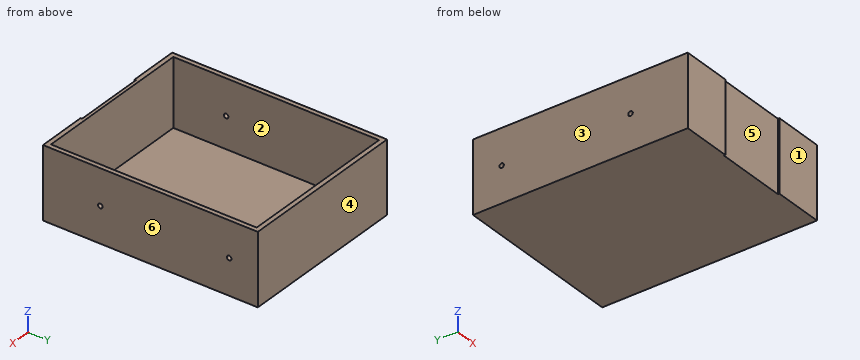
```python
from build123d import *

# Parameters (mm, degrees)
F0_W     = 113.645
F0_H     = 3.18
F0_W_2   = 3.175
F0_H_2   = 143.64
F0_W_3   = 3.18
F1_DEPTH = 50
F2_W     = 113.64
F2_H     = 143.64
F3_DEPTH = 47
F5_DEPTH = 120.001
F6_W     = 50
F6_H     = 50
F7_DEPTH = 1


with BuildPart() as f1:
    # F0 (on Top) → F1 (new body)
    with BuildSketch(Plane.XY):
        with Locations((-10.0610243238, 113.2212999272)):
            Rectangle(F0_W, F0_H)
        with Locations((-68.4710243238, 113.2212999272)):
            Rectangle(F0_W_2, F0_H)
        with Locations((-68.4710243238, 39.8112999272)):
            Rectangle(F0_W_2, F0_H_2)
        with Locations((-10.0610243238, -33.5987000728)):
            Rectangle(F0_W, F0_H)
        with Locations((48.3514756762, 39.8112999272)):
            Rectangle(F0_W_3, F0_H_2)
        with Locations((48.3514756762, -33.5987000728)):
            Rectangle(F0_W_3, F0_H)
        with Locations((48.3514756762, 113.2212999272)):
            Rectangle(F0_W_3, F0_H)
        with Locations((-68.4710243238, -33.5987000728)):
            Rectangle(F0_W_2, F0_H)
        with Locations((-10.0610243238, 39.8112999272)):
            Rectangle(F0_W, F0_H_2)
    extrude(amount=F1_DEPTH)

    # F2 (on face) → F3 (cut)
    with BuildSketch(Plane.XY.offset(50)):
        with Locations((-10.0585243238, 39.8112999272)):
            Rectangle(F2_W, F2_H)
    extrude(amount=-F3_DEPTH, mode=Mode.SUBTRACT)

    # F4 (on face) → F5 (cut, through all)
    with BuildSketch(Plane.YZ.offset(49.9414756762)):
        with BuildLine():
            ThreePointArc((6.4012999272, 25), (5.9355997093, 26.1242997821), (4.8112999272, 26.59))
            Line((4.8112999272, 26.59), (4.8112999272, 23.41))
            ThreePointArc((4.8112999272, 23.41), (5.9355997093, 23.8757002179), (6.4012999272, 25))
        make_face()
        with BuildLine():
            Line((4.8112999272, 23.41), (4.8112999272, 26.59))
            ThreePointArc((4.8112999272, 26.59), (3.2212999272, 25), (4.8112999272, 23.41))
        make_face()
        with BuildLine():
            ThreePointArc((96.4012999272, 25), (95.9355997093, 26.1242997821), (94.8112999272, 26.59))
            Line((94.8112999272, 26.59), (94.8112999272, 23.41))
            ThreePointArc((94.8112999272, 23.41), (95.9355997093, 23.8757002179), (96.4012999272, 25))
        make_face()
        with BuildLine():
            Line((94.8112999272, 23.41), (94.8112999272, 26.59))
            ThreePointArc((94.8112999272, 26.59), (93.2212999272, 25), (94.8112999272, 23.41))
        make_face()
    extrude(amount=-F5_DEPTH, mode=Mode.SUBTRACT)

    # F6 (on face) → F7 (cut)
    with BuildSketch(Plane.XZ.offset(35.1887000728)):
        with Locations((-10.0585243238, 25)):
            Rectangle(F6_W, F6_H)
    extrude(amount=-F7_DEPTH, mode=Mode.SUBTRACT)


solid = f1.part
```
Source: CAD feature listing. Evaluate the final solid. Frame: model axes, mm. Face numbers are marked on the shaded views. A direction names the side the tool comes from. Round coordinates to 2 decimals unless told otherwise and drop trailing zeros. Loops run counter-clockwise (first coordinate to the right, second up) from the corner with the lowest first, then second, coordinate; pieces in that order, holes last.
(1) Contact query for flat-ended pins moving along their axis: pin 1 Ø3 at (x, z) = (-20, 37.5) entering from -Y; pin 2 Ø3 at (x, y) = (-37.5, 30.5) entering from +Z. Output: stop coordinate, or through.
From the geometry:
pin 1: stops at y = -34.19
pin 2: stops at z = 3
(2) Section query A-A (z = 33). Output: boundary loops of the cut face in (x, y), and give its area (3 significant figures).
From the geometry:
outline: (-70.06, -35.19) - (-35.06, -35.19) - (-35.06, -34.19) - (14.94, -34.19) - (14.94, -35.19) - (49.94, -35.19) - (49.94, 114.81) - (-70.06, 114.81) - close; hole (-66.88, -32.01) - (46.76, -32.01) - (46.76, 111.63) - (-66.88, 111.63) - close
area: 1,630 mm2
(3) Section query B-B (y = -9.5). Output: boundary loops of the cut face in (x, z), and give its area (3 significant figures).
From the geometry:
outline: (-70.06, 0) - (49.94, 0) - (49.94, 50) - (46.76, 50) - (46.76, 3) - (-66.88, 3) - (-66.88, 50) - (-70.06, 50) - close
area: 659 mm2
(4) Section query C-C (x = -43). Output: boundary loops of the cut face in (y, z), and give its area (3 significant figures).
From the geometry:
outline: (-35.19, 0) - (114.81, 0) - (114.81, 50) - (111.63, 50) - (111.63, 3) - (-32.01, 3) - (-32.01, 50) - (-35.19, 50) - close
area: 749 mm2
(5) Pull-direction query (X, two-part tool) for the marked faces 3, 4, 5 and 6; classes: +X half, -X half, draft (parallel to the pull), parting line (faces both ways), or undercut.
From the geometry:
face 3: -X half
face 4: draft
face 5: undercut
face 6: +X half
(6) Access query for the marked faces 1 and 2. Directions: +Z, -Z, +X, -X, +Y, -Y. A direction counts if a zero-diameter tool reaches every point of the face in a straight line with its end or side. Return the directions, or none.
From the geometry:
face 1: +Z, -Z, +X, -X, -Y
face 2: +Z
(7) Material intervals for probe 1 along X at (y, z) = (96, 10); probe 2 along Y at (x, z) = (-40.5, 29); probe 3 along Y at (x, z) = (-8.5, 15.5), sorted ascending.
From the geometry:
probe 1: x = -70.06 to -66.88, 46.76 to 49.94
probe 2: y = -35.19 to -32.01, 111.63 to 114.81
probe 3: y = -34.19 to -32.01, 111.63 to 114.81
